from build123d import *

# Parameters (mm, degrees)
F0_W     = 114.3
F0_H     = 114.3
F0_W_2   = 106.68
F0_H_2   = 106.68
F1_DEPTH = 3.81
F2_DEPTH = 12.7
F4_R     = 19.05
F5_DEPTH = 6.858


with BuildPart() as f1:
    # F0 (on Top) → F1 (new body)
    with BuildSketch(Plane.XY):
        Rectangle(F0_W, F0_H)
        Rectangle(F0_W_2, F0_H_2, mode=Mode.SUBTRACT)
        Rectangle(F0_W_2, F0_H_2)
    extrude(amount=F1_DEPTH)

    # F0 (on Top) → F2 (join)
    with BuildSketch(Plane.XY):
        Rectangle(F0_W, F0_H)
        Rectangle(F0_W_2, F0_H_2, mode=Mode.SUBTRACT)
    extrude(amount=F2_DEPTH)

    # F4 (on face) → F5 (cut)
    with BuildSketch(Plane.XY.offset(3.81)):
        Circle(F4_R)
    extrude(amount=-F5_DEPTH, mode=Mode.SUBTRACT)


solid = f1.part
Design review of the part built by this model. Coordinates are the model's own, in mm. A direction names the side the tool comes from. Give positions to 0.01 mm unless a question says otherwise; leave off trailing zeros. Loops run counter-clockwise (first coordinate to the right, second up) from the corner with the lowest first, then second, coordinate; pieces in that order, holes last. Notation, with made-up numbers: (78, 45) -> (131, 45) arc R32 cw to (131, 78) -> close; hole circle Ø3 at (34.25, 53). An arc over 180 degrees is marked (long way). One line per question, with ' | ' between items. Start each with the question number.
(1) For faces 1 (the face through (53.34, -1, 8)), 2 (the face through (-14, 14, 0)), list the 3-axis set-ups (+Z, -Z, +X, -X, +Y, -Y) from which the entire face can be reached by the end or side of a thin tool; tool diameter is ignored.
(2) For line 1 (Y direction, x = -47.5, z = 8.25); line 2 (Y direction, x = 0, z = 3.05), list the stretches that pass through material, from the lowest coordinate up.
(3) We need section C-C (z = 10). State the section outline as (x, y) points, and give its area (3 significant figures).
(4) Draft analysis for pull direction Y (two halves, no side actions). For faces 3 (the face through (-1, 57.15, 6)), 4 (the face through (-57.15, -1, 6)), 5 (the face through (-1, -57.15, 6)), 6 (the face through (-53.34, -1, 8)), state which applies: +Y half, -Y half, draft (parallel to the pull), parting line (faces both ways), or undercut.
(5) We need section D-D (x = -20.5). State the section outline as (y, z) points, and give its area (3 significant figures).
(6) Insertion check: P1, Ø5, axis at x = -4, y = 31, coming from the +Z side. The pin has a flat end and moves straight along its axis. Give the tip position at first contact, or say it passes through.
(7) We need section A-A (y = 0). State the section outline as (x, z) points, and give its area (3 significant figures).
The answers:
1) face 1: +Z | face 2: -Z, +X, -X, +Y, -Y
2) line 1: y = -57.15 to -53.34, 53.34 to 57.15 | line 2: y = -57.15 to -19.05, 19.05 to 57.15
3) outline: (-57.15, -57.15) -> (57.15, -57.15) -> (57.15, 57.15) -> (-57.15, 57.15) -> close; hole (-53.34, -53.34) -> (53.34, -53.34) -> (53.34, 53.34) -> (-53.34, 53.34) -> close | area: 1,680 mm^2
4) face 3: +Y half | face 4: draft | face 5: -Y half | face 6: undercut
5) outline: (-57.15, 0) -> (57.15, 0) -> (57.15, 12.7) -> (53.34, 12.7) -> (53.34, 3.81) -> (-53.34, 3.81) -> (-53.34, 12.7) -> (-57.15, 12.7) -> close | area: 503 mm^2
6) P1: stops at z = 3.81
7) outline: (-57.15, 0) -> (-19.05, 0) -> (-19.05, 3.81) -> (-53.34, 3.81) -> (-53.34, 12.7) -> (-57.15, 12.7) -> close; (19.05, 0) -> (57.15, 0) -> (57.15, 12.7) -> (53.34, 12.7) -> (53.34, 3.81) -> (19.05, 3.81) -> close | area: 358 mm^2
